from build123d import *

# Parameters (mm, degrees)
SKETCH1_W           = 16.5
SKETCH1_H           = 25
BOSS_EXTRUDE1_DEPTH = 1.6
SKETCH2_R           = 1.5
CUT_EXTRUDE1_DEPTH  = 16.062287343
SKETCH3_W           = 13.2
SKETCH3_H           = 9.9
BOSS_EXTRUDE2_DEPTH = 8.8
SKETCH4_R           = 1.75
BOSS_EXTRUDE3_DEPTH = 8.1
SKETCH5_W           = 8.2
SKETCH5_H           = 5.602380094
BOSS_EXTRUDE4_DEPTH = 4.3
SKETCH6_W           = 6
SKETCH6_H           = 4
BOSS_EXTRUDE5_DEPTH = 3.5


with BuildPart() as part:
    # Sketch1 → Boss-Extrude1 (new body)
    with BuildSketch(Plane.XY):
        Rectangle(SKETCH1_W, SKETCH1_H)
    extrude(amount=BOSS_EXTRUDE1_DEPTH)

    # Sketch2 → Cut-Extrude1 (cut, through all)
    with BuildSketch(Plane.XY.offset(1.6)):
        with Locations((-6.25, 10.5)):
            Circle(SKETCH2_R)
        with Locations((6.25, -10.5)):
            Circle(SKETCH2_R)
    extrude(amount=-CUT_EXTRUDE1_DEPTH, mode=Mode.SUBTRACT)

    # Sketch3 → Boss-Extrude2 (add)
    with BuildSketch(Plane.XY.offset(1.6)):
        with Locations((0.65, 2.45)):
            Rectangle(SKETCH3_W, SKETCH3_H)
    extrude(amount=BOSS_EXTRUDE2_DEPTH)

    # Sketch4 → Boss-Extrude3 (add)
    with BuildSketch(Plane(origin=(0, 7.4, 0), x_dir=(1, 0, 0), z_dir=(0, 1, 0))):
        with Locations((-2.95, -6)):
            Circle(SKETCH4_R)
        with Locations((4.25, -6)):
            Circle(SKETCH4_R)
    extrude(amount=BOSS_EXTRUDE3_DEPTH)

    # Sketch5 → Boss-Extrude4 (add)
    with BuildSketch(Plane.XY.offset(1.6)):
        with Locations((-2.05, -9.698809953)):
            Rectangle(SKETCH5_W, SKETCH5_H)
    extrude(amount=BOSS_EXTRUDE4_DEPTH)

    # Sketch6 → Boss-Extrude5 (add)
    with BuildSketch(Plane(origin=(0, -12.5, 0), x_dir=(-1, 0, 0), z_dir=(0, -1, 0))):
        with Locations((2.05, -3.6)):
            Rectangle(SKETCH6_W, SKETCH6_H)
    extrude(amount=BOSS_EXTRUDE5_DEPTH)


solid = part.part
For this review, take the finished solid that the model builds, in its own axes (mm). A direction names the side the tool comes from. Give positions to 0.01 mm unless a question says otherwise; leave off trailing zeros. Order: outer loops, then holes, each group sorted by start corner. A loop starts at its lowest first (then second) coordinate and runs counter-clockwise, first axis right, second up. Notation, with made-up numbers: (30.25, -26.75) - (50.25, -26.75) arc R19 cw to (50.25, -13.75) - close; hole circle Ø6 at (89, 21.25). An arc over 180 degrees is marked (long way). Answer as a JSON object with one key per item and string values. Group by question number.
Item 1: Take a section at A-A on y = 10.5. Give the boundary of the cut face in (x, z).
Item 2: Draft analysis for pull direction X (two halves, no side actions). For faces 1 (the flat face through (2.05, -10, 4)), 2 (the flat face through (1, 7.4, 6)), 3 (the flat face through (-8.25, 0, 1)), state which applies: pulls with the +X half, pulls with the -X half, needs draft (parallel to the pull), parting line crosses it, or undercut.
Item 3: Clearance check with flat-ended pins moving along their axes: pin 1 Ø2 at (x, z) = (3, 5) entering from -Y; pin 2 Ø6 at (y, z) = (-5, 7) entering from -X; pin 3 Ø2 at (x, z) = (-5, 8) entering from +Y. State where each tip first meets the part, or that it passes through.
Item 4: Take a section at D-D on x = 4.25. Give the boundary of the cut face in (y, z), and give its area (3 significant figures).
Item 5: Take a section at B-B on z = 3.5. Give the boundary of the cut face in (x, y).
Item 6: Machinability: for faces 4 (the flat face through (0.95, -14, 4)), 5 (the flat face through (-5.95, 2, 6)), 6 (the flat face through (-2, -14, 1.6)), 7 (the flat face through (-6.15, -10, 4)), which of the approach directions +Z, -Z, +X, -X, +Y, -Y give a long, thin tool a straight path to every point of the face, cutting with its end or side? Answer none if there is none.
Item 7: Wall thickness on line 1 along Y through (x, z) = (6.25, 0.9); line 2 along Y through (x, z) = (-0.25, 4.5); line 3 along Z through (x, y) = (-7.5, -12): over which ranges is each line inside the solid? List them lowest first.
Item 8: Take a section at C-C on y = -10.5. Give the boundary of the cut face in (x, z), and give its area (3 significant figures).
Reported:
{
 "1": {"outline": "(-8.25, 0) - (-7.75, 0) - (-7.75, 1.6) - (-8.25, 1.6) - close; (-4.75, 0) - (8.25, 0) - (8.25, 1.6) - (-4.75, 1.6) - close; circle Ø3.5 at (-2.95, 6); circle Ø3.5 at (4.25, 6)"},
 "2": {"face 1": "pulls with the +X half", "face 2": "undercut", "face 3": "pulls with the -X half"},
 "3": {"pin 1": "y = -12.5", "pin 2": "x = -6.15", "pin 3": "y = 7.4"},
 "4": {"outline": "(-12.5, 0) - (12.5, 0) - (12.5, 1.6) - (7.4, 1.6) - (7.4, 4.25) - (15.5, 4.25) - (15.5, 7.75) - (7.4, 7.75) - (7.4, 10.4) - (-2.5, 10.4) - (-2.5, 1.6) - (-12.5, 1.6) - close", "area": "155 mm^2"},
 "5": {"outline": "(-6.15, -12.5) - (-5.05, -12.5) - (-5.05, -16) - (0.95, -16) - (0.95, -12.5) - (2.05, -12.5) - (2.05, -6.9) - (-6.15, -6.9) - close; (-5.95, -2.5) - (7.25, -2.5) - (7.25, 7.4) - (-5.95, 7.4) - close"},
 "6": {"face 4": "+Z, -Z, +X, -Y", "face 5": "+Z, -X, +Y", "face 6": "-Z, +X, -X, -Y", "face 7": "+Z, -X, +Y, -Y"},
 "7": {"line 1": "-12.5 to -12, -9 to 12.5", "line 2": "-16 to -6.9, -2.5 to 7.4", "line 3": "0 to 1.6"},
 "8": {"outline": "(-8.25, 0) - (4.75, 0) - (4.75, 1.6) - (2.05, 1.6) - (2.05, 5.9) - (-6.15, 5.9) - (-6.15, 1.6) - (-8.25, 1.6) - close; (7.75, 0) - (8.25, 0) - (8.25, 1.6) - (7.75, 1.6) - close", "area": "56.9 mm^2"}
}
